Can you work these out from the drawing? Everything is in mm from the part's minimum corner. A direction names the side the tool comes from. Coordinates: 2 decimals unless noted, no trailing zeros. Loops run counter-clockwise (first coordinate to the right, second up) from the corner with the lowest first, then second, coordinate; pieces in that order, holes last. Notation, with made-up numbers: (60, 0.5) - (83, 0.5) arc R16 cw to (83, 11.5) - close; hole circle Ø1 at (-1.75, 29.25). An arc over 180 degrees is marked (long way). One line per question, with ' | ' between items. Start each with the question number.
1. Please list where these lines run through material, in increasing order: L1, parallel to X at y = 16, z = 70; L2, parallel to Z at x = 95, y = 23.5; L3, parallel to Z at x = 9, y = 41. Write a range as [from, to].
2. I'm going to push a flat-ended pin straight in: P1, Ø1, axis at x = 69.5, y = 42.5, coming from the +Z side. Where does the tip first touch, or does it pass through?
3. I want a section at B-B, the plane x = 129. Write out the boundary of the cut face in (y, z), then the cut area to 3 significant figures.
4. I want a section at C-C, the plane z = 38. Write out the boundary of the cut face in (x, y), then the cut area to 3 significant figures.
5. I want a section at A-A, the plane y = 25.5. Write out the boundary of the cut face in (x, z), then the cut area to 3 significant figures.
6. I want a section at D-D, the plane y = 14. Write out the boundary of the cut face in (x, z), then the cut area to 3 significant figures.
7. Which directions (+Z, -Z, +X, -X, +Y, -Y) give clear straight access to the entire face, cutting with the end or side of a thin tool? Please do the marked faces 1 and 2.
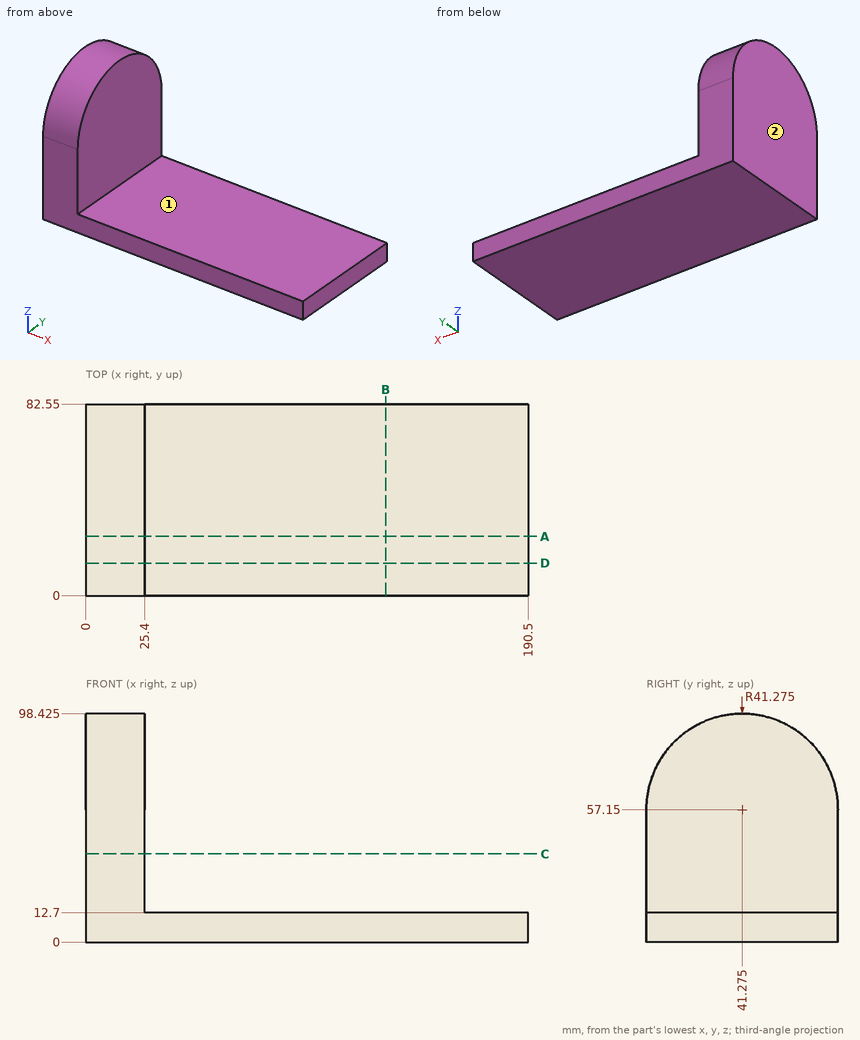
Results are:
1) L1: x = [0, 25.4] | L2: z = [0, 12.7] | L3: z = [0, 98.42]
2) P1: stops at z = 12.7
3) outline: (0, 0) - (82.55, 0) - (82.55, 12.7) - (0, 12.7) - close | area: 1,050 mm2
4) outline: (0, 0) - (25.4, 0) - (25.4, 82.55) - (0, 82.55) - close | area: 2,100 mm2
5) outline: (0, 0) - (190.5, 0) - (190.5, 12.7) - (25.4, 12.7) - (25.4, 95.29) - (0, 95.29) - close | area: 4,520 mm2
6) outline: (0, 0) - (190.5, 0) - (190.5, 12.7) - (25.4, 12.7) - (25.4, 88.13) - (0, 88.13) - close | area: 4,340 mm2
7) face 1: +Z, +X, +Y, -Y | face 2: +Z, -Z, -X, +Y, -Y
